Design review of the part built by this model. Coordinates are the model's own, in mm. A direction names the side the tool comes from. Give positions to 0.01 mm unless a question says otherwise; leave off trailing zeros. Order: outer loops, then holes, each group sorted by start corner. A loop starts at its lowest first (then second) coordinate and runs counter-clockwise, first axis right, second up. Notation, with made-up numbers: (-11, 44.5) -> (45, 44.5) arc R25 ccw to (45, 66.5) -> close; hole circle Ø7 at (32.25, 54.5). An arc over 180 degrees is marked (long way). One line per item, written item: value.
from build123d import *

# Parameters (mm, degrees)
F1_DEPTH = 8.25
F2_DEPTH = 7


# Not quite as in the source:
# - a feature names something its author has since deleted; it is built from what else it names


with BuildPart() as f1:
    # F0 (on Front) → F1 (new body, symmetric)
    with BuildSketch(Plane.XZ):
        with BuildLine():
            Line((-1.2599999983, 0.001106019), (-0.2481810163, 0.001106019))
            Line((-0.2481810241, 0.001106019), (-0.4941885147, 1.1379972147))
            Line((-0.4941885147, 1.1379972147), (-1.2832667135, 1.9140606746))
            Line((-1.2832667135, 1.9140606746), (-2.2277169394, 2.3196199825))
            Line((-2.2277169394, 2.3196199825), (-3.3833966788, 2.3196199825))
            Line((-3.3833966788, 2.3196199825), (-4.2535923825, 1.9888198258))
            Line((-4.2535923825, 1.9888198258), (-5.0546050044, 1.1417629963))
            Line((-5.0546050044, 1.1417629963), (-5.7481810085, 0.001106019))
            Line((-5.7481810085, 0.001106019), (-4.0599999983, 0.001106019))
            ThreePointArc((-4.0599999983, 0.001106019), (-2.6599999983, 1.401106019), (-1.2599999983, 0.001106019))
        make_face()
        with BuildLine():
            ThreePointArc((-1.0547499373, -1.9445495701), (-0.4578133732, -1.0519999951), (-0.2481810085, 0.001106019))
            Line((-0.2481810163, 0.001106019), (-1.2599999983, 0.001106019))
            ThreePointArc((-1.2599999983, 0.001106019), (-2.6599999983, -1.398893981), (-4.0599999983, 0.001106019))
            Line((-4.0599999983, 0.001106019), (-5.7481810085, 0.001106019))
            ThreePointArc((-5.7481810085, 0.001106019), (-4.0512870227, -2.5392616163), (-1.0547499373, -1.9445495701))
        make_face()
        with BuildLine():
            Line((-4.0599999966, -4.9463636499), (-1.0547499373, -1.9445495701))
            ThreePointArc((-1.0547499373, -1.9445495701), (-4.0512870227, -2.5392616163), (-5.7481810085, 0.001106019))
            Line((-5.7481810085, 0.001106019), (-5.9999999983, -1.1473703696))
            Line((-5.9999999983, -1.1473703696), (-5.9999999983, -4.8066070303))
            Line((-5.9999999983, -4.8066070303), (-5.9999999983, -6.0053556226))
            Line((-5.9999999983, -6.0053556226), (-5.1202041279, -6.0053556226))
            Line((-5.1202041279, -6.0053556226), (-4.0599999966, -4.9463636499))
        make_face()
        Polygon((-4.0599999966, -6.0053556226), (-4.0599999966, -4.9463636499), (-5.1202041279, -6.0053556226), align=None)
    extrude(amount=F1_DEPTH, both=True)

    # F0 (on Front) → F2 (join)
    with BuildSketch(Plane.XZ):
        with BuildLine():
            Line((-1.2832667135, 1.9140606746), (-0.4941885147, 1.1379972147))
            ThreePointArc((-0.4941885147, 1.1379972147), (-3.5797825225, 2.6889005943), (-5.7481810085, 0.001106019))
            Line((-5.7481810085, 0.001106019), (-5.0546050044, 1.1417629963))
            Line((-5.0546050044, 1.1417629963), (-4.2535923825, 1.9888198258))
            Line((-4.2535923825, 1.9888198258), (-3.3833966788, 2.3196199825))
            Line((-3.3833966788, 2.3196199825), (-2.2277169394, 2.3196199825))
            Line((-2.2277169394, 2.3196199825), (-1.2832667135, 1.9140606746))
        make_face()
        Polygon((-5.9999999983, -1.1473703696), (-5.7481810085, 0.001106019), (-6, 0.001106019), align=None)
        Polygon((-4.0599999966, -14.9466558945), (-4.0599999966, -8.645166643), (-5.9999999983, -8.645166643), (-5.9999999983, -30), (-4.4599999966, -19.4339305162), align=None)
        Polygon((-4.0599999966, -6.0053556226), (-5.1202041279, -6.0053556226), (-6, -6.8841456016), (-5.9999999983, -8.645166643), (-4.0599999966, -8.645166643), align=None)
        Polygon((-6, -6.8841456016), (-5.1202041279, -6.0053556226), (-5.9999999983, -6.0053556226), align=None)
    extrude(amount=F2_DEPTH)


solid = f1.part
Item 1: Machinability: for faces 1 (the flat face through (-3.812, -7.634, 2.157)), 2 (the flat face through (-1.749, -7.634, 2.114)), 3 (the flat face through (-3.812, 4.067, 2.157)), 4 (the flat face through (-1.749, 4.067, 2.114)), which of the approach directions +Z, -Z, +X, -X, +Y, -Y give a long, thin tool a straight path to every point of the face, cutting with its end or side? Answer none if there is none.
Returned:
face 1: +Z, -X, -Y
face 2: +Z, +X, -Y
face 3: +Z, -X, +Y
face 4: +Z, +X, +Y
Item 2: Clearance check with flat-ended pins moving along their axes: P1, Ø3, axis at x = -5, y = -1, coming from the +Z side; P2, Ø1.5, axis at x = -2, y = -5, coming from the -Z side; P3, Ø2, axis at x = -5.5, z = -22, coming from the +Y side. State where each tip first meets the part, or that it passes through.
Returned:
P1: z = 2.7
P2: z = -3.64
P3: y = 0
Item 3: Add section A-A on y = -1.25. Give the boundary of the cut face in (x, z).
Returned:
outline: (-6, -30) -> (-4.46, -19.43) -> (-4.06, -14.95) -> (-4.06, -4.95) -> (-1.05, -1.94) arc R2.75 ccw to (-0.25, 0) -> (-0.49, 1.14) arc R2.75 ccw to (-5.75, 0) -> (-6, 0) -> close; hole circle Ø2.8 at (-2.66, 0)
Item 4: Add section B-B on z = -0.5. Give the boundary of the cut face in (x, y).
Returned:
outline: (-6, -7) -> (-5.86, -7) -> (-5.86, -8.25) -> (-3.97, -8.25) -> (-3.97, 8.25) -> (-5.86, 8.25) -> (-5.86, 0) -> (-6, 0) -> close; (-1.35, -8.25) -> (-0.29, -8.25) -> (-0.29, 8.25) -> (-1.35, 8.25) -> close
Item 5: To check wall thickness, follow line 1 along X through (y, z) = (-4.5, -13); line 2 along Y through (x, z) = (-5.3, -23); line 3 along Z through (x, y) = (-2.66, -0.5). State the ranges of each line that lie inside material, in increasing order. Write a range as from..to.
Returned:
line 1: -6..-4.06
line 2: -7..0
line 3: -3.55..-1.4, 1.4..2.73
Item 6: Add section C-C on x = -2.9. Give the boundary of the cut face in (y, z).
Returned:
outline: (-8.25, -3.79) -> (8.25, -3.79) -> (8.25, -1.38) -> (-8.25, -1.38) -> close; (-8.25, 1.38) -> (8.25, 1.38) -> (8.25, 2.32) -> (0, 2.32) -> (0, 2.75) -> (-7, 2.75) -> (-7, 2.32) -> (-8.25, 2.32) -> close
Item 7: Add section D-D on y = 7.25. Give the boundary of the cut face in (x, z).
Returned:
outline: (-6, -6.01) -> (-4.06, -6.01) -> (-4.06, -4.95) -> (-1.05, -1.94) arc R2.75 ccw to (-0.25, 0) -> (-0.49, 1.14) -> (-1.28, 1.91) -> (-2.23, 2.32) -> (-3.38, 2.32) -> (-4.25, 1.99) -> (-5.05, 1.14) -> (-5.75, 0) -> (-6, -1.15) -> close; hole circle Ø2.8 at (-2.66, 0)
